Design review of the part built by this model. Coordinates are the model's own, in mm. A direction names the side the tool comes from. Coordinates: 2 decimals unless noted, no trailing zeros. Order: outer loops, then holes, each group sorted by start corner. A loop starts at its lowest first (then second) coordinate and runs counter-clockwise, first axis right, second up.
from build123d import *

# Parameters (mm, degrees)
FILLET1_R   = 0.25
FILLET2_R   = 0.6
HEX_2_DEPTH = 2.5


with BuildPart() as part:
    # BodySke → Base-Revolve (revolve)
    with BuildSketch(Plane.XY):
        Polygon((0, 0), (0, 5), (4, 5), (4, 3), (23.4455, 3), (24, 2.4455), (24, 0), align=None)
    revolve(axis=Axis((-31.75, 0, 0), (1, 0, 0)))

    # Fillet1
    fillet1_edges = [part.edges().sort_by_distance(p)[0] for p in [
        (4, -3, 0),
    ]]
    fillet(fillet1_edges, radius=FILLET1_R)

    # Fillet2
    fillet2_edges = [part.edges().sort_by_distance(p)[0] for p in [
        (0, -5, 0),
    ]]
    fillet(fillet2_edges, radius=FILLET2_R)

    # HexSke → Hex 2 (cut)
    with BuildSketch(Plane(origin=(0, 0, 0), x_dir=(0, 0.5, 0.866025404), z_dir=(-1, 0, 0))):
        Polygon((1.443375673, 2.5), (-1.443375673, 2.5), (-2.886751346, 0), (-1.443375673, -2.5), (1.443375673, -2.5), (2.886751346, 0), align=None)
    extrude(amount=-HEX_2_DEPTH, mode=Mode.SUBTRACT)

    # PilotSke → Hex-PreBroach (revolve, cut)
    with BuildSketch(Plane.XY):
        Polygon((0, 2.5), (2.5, 2.5), (3.077350269, 1.5), (5, 1.5), (5.866025404, 0), (0, 0), align=None)
    revolve(axis=Axis((0, 0, 0), (1, 0, 0)), mode=Mode.SUBTRACT)


solid = part.part
1. Mouldability with a two-part tool opening along Z and no side actions: class faces 4 (the flat face through (1, 0, 2.5)), 5 (the flat face through (24, 0, 0)), 6 (the cylindrical face through (2.32, -1.08, -4.88)) as pulls with the +Z half, pulls with the -Z half, needs draft (parallel to the pull), parting line crosses it, or undercut.
2. Add section A-A (x = 15.5). Give the boundary of the cut face in (y, z).
3. Insertion check: pin 1 (3 mm diameter, centred on x = 1, y = -0.5, fed in from +Z); pin 2 (1.4 mm diameter, centred on y = -0.5, z = -1.5, fed in from -X); pin 3 (6 mm diameter, centred on x = 3, y = -3.5, fed in from -Z); pin 4 (1.5 mm diameter, centred on x = 15, y = -2.5, fed in from +Z). Each pin has a flat end and moves straight along its axis. Give the tip position at first contact, or say it passes through.
4. For faces 1 (the flat face through (1.232, 2.155, 1.268)), 2 (the flat face through (0, -2, -2)), 3 (the cylindrical face through (14, -3, 0)), list the 3-axis set-ups (+Z, -Z, +X, -X, +Y, -Y) from which the entire face can be reached by the end or side of a thin tool; tool diameter is ignored.
5. To check wall thickness, follow line 1 (Z direction, x = 4.45, y = 0); line 2 (X direction, y = -3.25, z = -2); line 3 (Z direction, x = 3.5, y = -0.5). State the ranges of each line that lie inside material, in increasing order.
Solution:
1. face 4: undercut
1. face 5: needs draft
1. face 6: parting line crosses it
2. outline: circle Ø6 at (0, 0)
3. pin 1: stops at z = 5
3. pin 2: stops at x = 2.63
3. pin 3: stops at z = -4.97
3. pin 4: stops at z = 2.44
4. face 1: -X
4. face 2: +Z, -Z, -X, +Y, -Y
4. face 3: +X
5. line 1: z = -3 to -1.5, 1.5 to 3
5. line 2: x = 0 to 4
5. line 3: z = -4.97 to -1.41, 1.41 to 4.97
